The model under review builds one solid part; all positions refer to its coordinate system, in mm. Face numbers are marked on the shaded views. Coordinates: 2 decimals unless noted, no trailing zeros. Order: outer loops, then holes, each group sorted by start corner. A loop starts at its lowest first (then second) coordinate and runs counter-clockwise, first axis right, second up. Notation, with made-up numbers: (84, 59.5) - (128, 59.5) arc R25 cw to (128, 97.5) - close; hole circle Ø10 at (66, 61). An arc over 180 degrees is marked (long way). Answer in a Markdown table with one row per item.
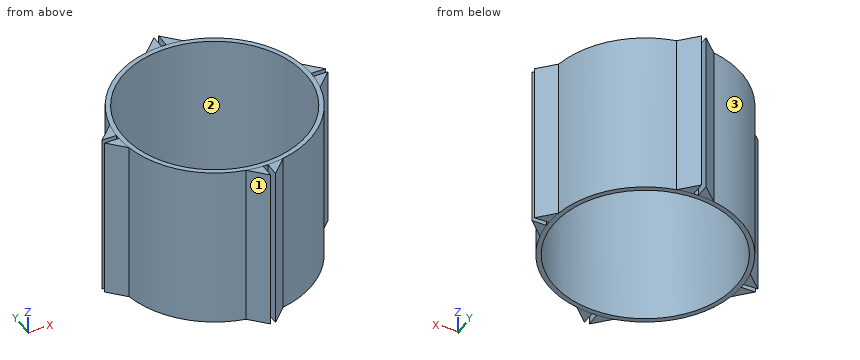
Autodesk Fusion 360 part; units mm, degrees
sketch "Sketch1" plane through (0, 0, 0) normal (0, 0, 1) x (1, 0, 0)
  circle A0 centre (0, 0) radius 38.5
  circle A1 centre (0, 0) radius 40.5
  line L0 (40.497, 0.49) -> (46.497, 0.49)
  line L1 (46.497, 0.49) -> (39.8697, 7.1173)
  line L2 (46.497, 0.49) -> (37.1246, 0.49) construction
  line L3 (46.497, 0.49) -> (46.497, -1.51) construction
  line L4 (37.1246, 0.49) -> (37.1246, -1.51) construction
  line L5 (37.1246, -1.51) -> (40.4718, -1.51) construction
  line L6 (40.4718, -1.51) -> (46.4718, -1.51)
  line L7 (46.4718, -1.51) -> (39.6294, -8.3525)
  line L8 (-1, 37) -> (1, 37) construction
  line L9 (1, 37) -> (1, 40.4877) construction
  line L10 (-1, 37) -> (-1, 40.4877) construction
  line L11 (-1, 40.4877) -> (-1, 46.4877)
  line L12 (-1, 46.4877) -> (-7.7327, 39.7549)
  line L13 (1, 40.4877) -> (1, 46.4877)
  line L14 (1, 46.4877) -> (7.7327, 39.7549)
  line L15 (-35, 1) -> (-35, -1) construction
  line L16 (-35, -1) -> (-40.4877, -1) construction
  line L17 (-35, 1) -> (-40.4877, 1) construction
  line L18 (-40.4877, -1) -> (-46.4877, -1)
  line L19 (-46.4877, -1) -> (-39.7549, -7.7327)
  line L20 (-40.4877, 1) -> (-46.4877, 1)
  line L21 (-46.4877, 1) -> (-39.7549, 7.7327)
  line L22 (-1, -37.5) -> (1, -37.5) construction
  line L23 (1, -37.5) -> (1, -40.4877) construction
  line L24 (-1, -37.5) -> (-1, -40.4877) construction
  line L25 (-1, -40.4877) -> (-1, -46.4877)
  line L26 (-1, -46.4877) -> (-7.7327, -39.7549)
  line L27 (1, -40.4877) -> (1, -46.4877)
  line L28 (1, -46.4877) -> (7.7327, -39.7549)
  dimension "d5" = 77
  dimension "d6" = 81
  dimension "d7" = 81
  dimension "d8" = 6
  dimension "d9" = 45
  dimension "d10" = 2
  dimension "d11" = 2
  dimension "d12" = 6
  dimension "d13" = 45
  dimension "d14" = 2
  dimension "d15" = 6
  dimension "d16" = 45
  dimension "d17" = 6
  dimension "d18" = 45
  dimension "d19" = 2
  dimension "d20" = 6
  dimension "d21" = 45
  dimension "d22" = 6
  dimension "d23" = 45
  dimension "d24" = 2
  dimension "d25" = 6
  dimension "d26" = 45
  dimension "d27" = 6
  dimension "d28" = 45
extrude "Extrude1" add sketch "Sketch1" along normal blind 70
equation "ytredim = 77 mm"
equation "lengdeholder = 6 mm"
equation "breddeholder = 2 mm"
equation "gradholder = 45 deg"
equation "d5 = ytredim"
equation "d6 = ytredim + 4 mm"
equation "d8 = lengdeholder"
equation "d9 = gradholder"
equation "d10 = breddeholder"
equation "d11 = breddeholder"
equation "d12 = lengdeholder"
equation "d13 = gradholder"
equation "d14 = breddeholder"
equation "d15 = lengdeholder"
equation "d16 = gradholder"
equation "d17 = lengdeholder"
equation "d18 = gradholder"
equation "d19 = breddeholder"
equation "d20 = lengdeholder"
equation "d21 = gradholder"
equation "d22 = lengdeholder"
equation "d23 = gradholder"
equation "d24 = breddeholder"
equation "d25 = lengdeholder"
equation "d26 = gradholder"
equation "d27 = lengdeholder"
equation "d28 = gradholder"
Item 1: Clearance check with flat-ended pins moving along their axes: pin 1 Ø3 at (y, z) = (-25, 38) entering from +X; pin 2 Ø5 at (x, z) = (42.5, 39.5) entering from +Y; pin 3 Ø3 at (x, z) = (-44.5, 27.5) entering from -Y; pin 4 Ø2 at (x, y) = (20.5, -34.5) entering from -Z. State where each tip first meets the part, or that it passes through.
Check values:
| item | result |
|---|---|
| pin 1 | x = 32.98 |
| pin 2 | y = 6.99 |
| pin 3 | y = -4.49 |
| pin 4 | z = 0 |
Item 2: We need section A-A, the plane y = -13. Write out the cut boundary in (x, z).
Check values:
| item | result |
|---|---|
| outline | (-38.36, 0) - (-36.24, 0) - (-36.24, 70) - (-38.36, 70) - close; (36.24, 0) - (38.36, 0) - (38.36, 70) - (36.24, 70) - close |
Item 3: To check wall thickness, follow line 1 (Y direction, x = 0, z = 25.5); line 2 (X direction, y = 31, z = 54.5); line 3 (Y direction, x = -24, z = 57). State the ranges of each line that lie inside material, in increasing order. Write a range as from..to.
Check values:
| item | result |
|---|---|
| line 1 | -40.5..-38.5, 38.5..40.5 |
| line 2 | -26.06..-22.83, 22.83..26.06 |
| line 3 | -32.62..-30.1, 30.1..32.62 |
Item 4: We need section B-B, the plane x = -36.5. Write out the cut boundary in (y, z), then the cut area to 3 significant figures.
Check values:
| item | result |
|---|---|
| outline | (-17.55, 0) - (-12.25, 0) - (-12.25, 70) - (-17.55, 70) - close; (12.25, 0) - (17.55, 0) - (17.55, 70) - (12.25, 70) - close |
| area | 742 mm^2 |
Item 5: We need section C-C, the plane z = 17. Write out the cut boundary in (x, y), then the cut area to 3 significant figures.
Check values:
| item | result |
|---|---|
| outline | (-46.49, -1) - (-39.75, -7.73) arc R40.5 ccw to (-7.73, -39.75) - (-1, -46.49) - (-1, -40.49) arc R40.5 ccw to (1, -40.49) - (1, -46.49) - (7.73, -39.75) arc R40.5 ccw to (39.63, -8.35) - (46.47, -1.51) - (40.47, -1.51) arc R40.5 ccw to (40.5, 0.49) - (46.5, 0.49) - (39.87, 7.12) arc R40.5 ccw to (7.73, 39.75) - (1, 46.49) - (1, 40.49) arc R40.5 ccw to (-1, 40.49) - (-1, 46.49) - (-7.73, 39.75) arc R40.5 ccw to (-39.75, 7.73) - (-46.49, 1) - (-40.49, 1) arc R40.5 ccw to (-40.49, -1) - close; hole circle Ø77 at (0, 0) |
| area | 653 mm^2 |
Item 6: Mouldability with a two-part tool opening along Y and no side actions: class the marked faces 1, 2 and 3 as +Y half, -Y half, draft (parallel to the pull), parting line (faces both ways), or undercut.
Check values:
| item | result |
|---|---|
| face 1 | -Y half |
| face 2 | undercut |
| face 3 | +Y half |
